The figure shows three views and two pictorial views of one solid part (mm, origin at its lowest corner). Answer the questions. A direction names the side the tool comes from. Give positions to 0.01 mm unless a question says otherwise; leave off trailing zeros. Loops run counter-clockwise (first coordinate to the right, second up) from the corner with the lowest first, then second, coordinate; pieces in that order, holes last. Notation, with made-up numbers: (16, 74.5) - (59, 74.5) arc R18 ccw to (59, 91.5) - close; hole circle Ø8 at (-34, 15). An arc over 180 degrees is marked (long way). One line per question, with ' | ' between items.
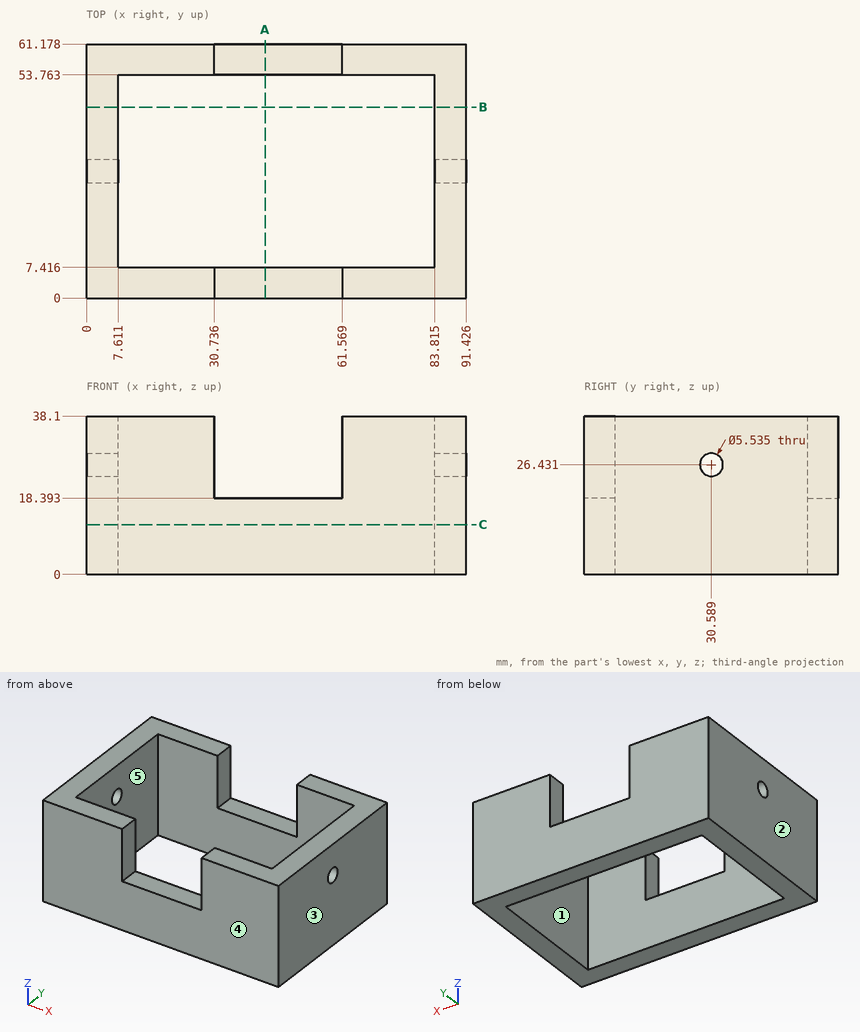
1. Which of the six approach directions +Z, -Z, +X, -X, +Y, -Y give full straight-line access (tool end or side, diameter ignored) to the marked faces 1 and 2?
Evaluation:
face 1: +Z, -Z | face 2: +Z, -Z, -X, +Y, -Y
2. Determine the mould class of the marked faces 3, 4 and 5 for opening direction Y: +Y half, -Y half, draft (parallel to the pull), parting line (faces both ways), or undercut.
Evaluation:
face 3: draft | face 4: -Y half | face 5: undercut
3. Find section A-A on x = 43. Write down the section's boundary in (y, z) (1 decimal), then the cut area to 3 significant figures.
Evaluation:
outline: (0, 0) - (7.4, 0) - (7.4, 18.4) - (0, 18.4) - close; (53.8, 0) - (61.2, 0) - (61.2, 18.4) - (53.8, 18.4) - close | area: 273 mm2
4. Flat-ended cylindrical pins translate along their axes: pin 1 (5 mm diameter, centred on y = 20.5, z = 17, fed in from -X); pin 2 (5 mm diameter, centred on y = 30.59, z = 26.43, fed in from +X); pin 3 (8 mm diameter, centred on x = 53.5, y = 55.5, fed in from +Z). Find the tip coordinate at first contact, or state that the pin passes through.
Evaluation:
pin 1: x = 0 | pin 2: through | pin 3: z = 18.39
5. Find section C-C on z = 12. Write down the section's boundary in (x, y) (1 decimal).
Evaluation:
outline: (0, 0) - (91.4, 0) - (91.4, 61.2) - (0, 61.2) - close; hole (7.6, 7.4) - (83.8, 7.4) - (83.8, 53.8) - (7.6, 53.8) - close
6. Consider L1, parallel to X at y = 58, z = 23 (1 decimal); L2, parallel to Y at x = 62.5, z = 10 (1 decimal); L3, parallel to X at y = 43.5, z = 20 (1 decimal). Determine where each line is inside the solid, lowest interval first.
Evaluation:
L1: 0 to 30.7, 61.6 to 91.4 | L2: 0 to 7.4, 53.8 to 61.2 | L3: 0 to 7.6, 83.8 to 91.4
7. Find section B-B on y = 46. Write down the section's boundary in (x, z) (1 decimal), then the cut area to 3 significant figures.
Evaluation:
outline: (0, 0) - (7.6, 0) - (7.6, 38.1) - (0, 38.1) - close; (83.8, 0) - (91.4, 0) - (91.4, 38.1) - (83.8, 38.1) - close | area: 580 mm2
